Verification items for the finished model (mm, model axes). A direction names the side the tool comes from. Give positions to 0.01 mm unless a question says otherwise; leave off trailing zeros. Order: outer loops, then holes, each group sorted by start corner. A loop starts at its lowest first (then second) coordinate and runs counter-clockwise, first axis right, second up. Notation, with made-up numbers: M -38.75,18.25 L 19.25,18.25 A36 cw 19.25,57.25 Z; hole C 12.5,63 d2. An arc over 180 degrees is marked long. Answer as a JSON object with one key per item and string values.
```python
from build123d import *

# Parameters (mm, degrees)
CUT_EXTRUDE1_DEPTH  = 5
CUT_EXTRUDE11_DEPTH = 5


with BuildPart() as part:
    # Sketch1 → Revolve1 (revolve)
    with BuildSketch(Plane(origin=(0, 0, 0), x_dir=(1, 0, 0), z_dir=(0, 1, 0))):
        Polygon((0, 0), (0, -265), (0, -340), (16, -340), (16, -295), (17, -295), (17, -245), (20, -245), (20, -95), (16, -95), (16, -45), (15, -45), (15, 0), align=None)
    revolve(axis=Axis((0, 0, 0), (0, 0, 1)))

    # Sketch3 → Cut-Extrude1 (cut)
    with BuildSketch(Plane(origin=(2.233419524, 16, 45), x_dir=(0, 0, -1), z_dir=(0, -1, 0))):
        with BuildLine():
            Line((-10, 2.766580476), (-40, 2.766580476))
            ThreePointArc((-40, 2.766580476), (-45, -2.233419524), (-40, -7.233419524))
            Line((-40, -7.233419524), (-10, -7.233419524))
            ThreePointArc((-10, -7.233419524), (-5, -2.233419524), (-10, 2.766580476))
        make_face()
    extrude(amount=CUT_EXTRUDE1_DEPTH, mode=Mode.SUBTRACT)

    # Sketch31 → Cut-Extrude11 (cut)
    with BuildSketch(Plane(origin=(1.137793825, 20, 245), x_dir=(0, 0, 1), z_dir=(0, -1, 0))):
        with BuildLine():
            Line((-30, 7.137793825), (-90, 7.137793825))
            ThreePointArc((-90, 7.137793825), (-96, 1.137793825), (-90, -4.862206175))
            Line((-90, -4.862206175), (-30, -4.862206175))
            ThreePointArc((-30, -4.862206175), (-24, 1.137793825), (-30, 7.137793825))
        make_face()
    extrude(amount=CUT_EXTRUDE11_DEPTH, mode=Mode.SUBTRACT)


solid = part.part
```
Q1. Gauge pin test, flat ends, axial feed: pin 1 Ø9.5 at (x, z) = (1, 174) entering from +Y; pin 2 Ø1.3 at (y, z) = (13.5, 64) entering from +X; pin 3 Ø1.5 at (y, z) = (-12, 208.5) entering from -X. Record the tip position at first contact, or that the pin passes through.
Resolved:
{"pin 1": "stops at y = 15", "pin 2": "stops at x = 9.53", "pin 3": "stops at x = -16.54"}
Q2. Release check for a two-part mould opening along Z. For faces 1 (the face through (0, 11, 70)), 2 (the face through (9.139, 14.334, 269.65)), 3 (the face through (-8.98, 13.43, 95)) record: +Z half, -Z half, draft (parallel to the pull), parting line (faces both ways), or undercut.
Resolved:
{"face 1": "undercut", "face 2": "draft", "face 3": "-Z half"}
Q3. Tool access check on faces 4 (the face through (0, 18, 149)), 5 (the face through (0, 0, 340)), 6 (the face through (-14.985, 0.66, 22.185)), 7 (the face through (9, -15, 245)). Record the directions out of +Z, -Z, +X, -X, +Y, -Y that give a thin tool (end or side, any length) a straight path to the whole face; none if there is none.
Resolved:
{"face 4": "+Y", "face 5": "+Z, +X, -X, +Y, -Y", "face 6": "-Z", "face 7": "+Z"}
Q4. Section check D-D on y = -11. Record the cut outline in (x, z), then the cut area to 3 significant figures.
Resolved:
{"outline": "M -16.7,95 L -11.62,95 L -11.62,45 L -10.2,45 L -10.2,0 L 10.2,0 L 10.2,45 L 11.62,45 L 11.62,95 L 16.7,95 L 16.7,245 L 12.96,245 L 12.96,295 L 11.62,295 L 11.62,340 L -11.62,340 L -11.62,295 L -12.96,295 L -12.96,245 L -16.7,245 Z", "area": "9,430 mm²"}
Q5. Section check A-A on x = 0. Record the cut outline in (y, z), then the cut area to 3 significant figures.
Resolved:
{"outline": "M -20,95 L -16,95 L -16,45 L -15,45 L -15,0 L 15,0 L 15,45 L 16,45 L 16,50 L 11,50 L 11,90 L 16,90 L 16,95 L 20,95 L 20,149 L 15,149 L 15,221 L 20,221 L 20,245 L 17,245 L 17,295 L 16,295 L 16,340 L -16,340 L -16,295 L -17,295 L -17,245 L -20,245 Z", "area": "11,500 mm²"}
Q6. Material ranges on L1, parallel to Z at x = 10, y = -16.5; L2, parallel to Y at x = 10.5, z = 125; L3, parallel to Z at x = 4, y = 14, recorded low to high.
Resolved:
{"L1": "z = 95 to 245", "L2": "y = -17.02 to 17.02", "L3": "z = 0 to 52, 88 to 340"}
Q7. Section check C-C on z = 103. Record the cut outline in (x, y).
Resolved:
{"outline": "C 0,0 d40"}
Q8. Section check B-B on y = 5.5. Record the cut outline in (x, z).
Resolved:
{"outline": "M -19.23,95 L -15.02,95 L -15.02,45 L -13.96,45 L -13.96,0 L 13.96,0 L 13.96,45 L 15.02,45 L 15.02,95 L 19.23,95 L 19.23,245 L 16.09,245 L 16.09,295 L 15.02,295 L 15.02,340 L -15.02,340 L -15.02,295 L -16.09,295 L -16.09,245 L -19.23,245 Z"}
